Verification items for the finished model (mm, model axes). Round coordinates to 2 decimals unless told otherwise and drop trailing zeros. Write each loop counter-clockwise with the first axis right and the second up, starting at its lowest first coordinate (ties: lowest second). Pieces come first, ordered by that corner, then holes. Notation, with made-up numbers: (4.5, -22) - (31.5, -22) arc R16 ccw to (31.5, -4) - close; hole circle Ø8 at (-13, 89.25). An arc over 180 degrees is marked (long way). Answer as a JSON object with one key per item and string values.
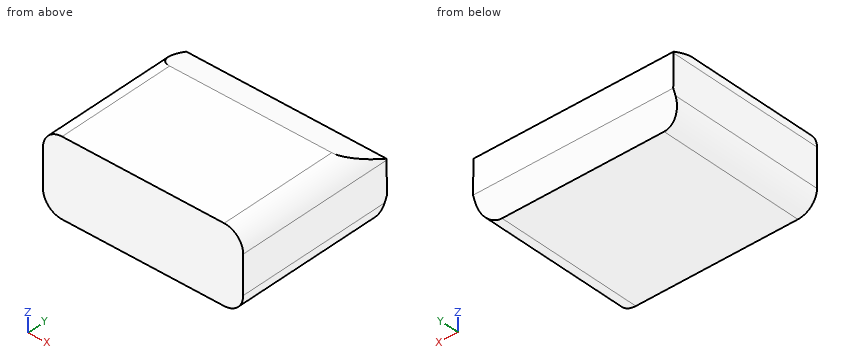
```python
from build123d import *

# Parameters (mm, degrees)
SKETCH1_W           = 105
SKETCH1_H           = 90
BOSS_EXTRUDE1_DEPTH = 40
FILLET5_R           = 10.000000066
FILLET6_R           = 10.000000066
FILLET7_R           = 10.000000066
FILLET8_R           = 10.000000066
CHAMFER14_SIZE      = 27.54
CHAMFER14_SIZE_2    = 12.3
CHAMFER15_SIZE      = 415.05734945
CHAMFER15_SIZE_2    = 7.46


with BuildPart() as part:
    # Sketch1 → Boss-Extrude1 (new body)
    with BuildSketch(Plane.XY):
        with Locations((7.000234735, -13.857374392)):
            Rectangle(SKETCH1_W, SKETCH1_H)
    extrude(amount=BOSS_EXTRUDE1_DEPTH)

    # Fillet5
    fillet5_edges = [part.edges().sort_by_distance(p)[0] for p in [
        (59.500234735, -13.857374392, 40),
    ]]
    fillet(fillet5_edges, radius=FILLET5_R)

    # Fillet6
    fillet6_edges = [part.edges().sort_by_distance(p)[0] for p in [
        (-45.499765265, -13.857374392, 40),
    ]]
    fillet(fillet6_edges, radius=FILLET6_R)

    # Fillet7
    fillet7_edges = [part.edges().sort_by_distance(p)[0] for p in [
        (59.500234735, -13.857374392, 0),
    ]]
    fillet(fillet7_edges, radius=FILLET7_R)

    # Fillet8
    fillet8_edges = [part.edges().sort_by_distance(p)[0] for p in [
        (-45.499765265, -13.857374392, 0),
    ]]
    fillet(fillet8_edges, radius=FILLET8_R)

    # Chamfer14
    # the kernel refuses this chamfer: 27.54, 12.3 mm, written as the material it takes off along each edge
    with BuildSketch(Plane(origin=(-106.873201315, 31.142625608, 0), x_dir=(0, 0.015735241575877565, 0.99987619342224), z_dir=(1, 0, 0))) as chamfer14_piece_1:
        Polygon((CHAMFER14_SIZE * 0.999876193422, CHAMFER14_SIZE * 0.0157352415759), (-CHAMFER14_SIZE_2 * 0.0157352415759, CHAMFER14_SIZE_2 * 0.999876193422), (0, 0), align=None)
    extrude(amount=227.7468721, mode=Mode.SUBTRACT)
    with BuildSketch(Plane(origin=(-106.873201315, 31.142625608, 40), x_dir=(0, 0.07864976650804911, -0.9969023092701859), z_dir=(1, 0, 0))) as chamfer14_piece_2:
        Polygon((CHAMFER14_SIZE_2 * 0.99690230927, -CHAMFER14_SIZE_2 * 0.078649766508), (-CHAMFER14_SIZE * 0.078649766508, -CHAMFER14_SIZE * 0.99690230927), (0, 0), align=None)
    extrude(amount=227.7468721, mode=Mode.SUBTRACT)

    # Chamfer15
    # the kernel refuses this chamfer: 415.05734945, 7.46 mm, written as the material it takes off along each edge
    with BuildSketch(Plane(origin=(-1124.643578574, 31.142625608, 27.7), x_dir=(0, 0.0006265203958835344, -0.9999998037360776), z_dir=(1, 0, 0))) as chamfer15_piece_1:
        Polygon((CHAMFER15_SIZE * 0.999999803737, -CHAMFER15_SIZE * 0.000626520395884), (-CHAMFER15_SIZE_2 * 0.408370910279, -CHAMFER15_SIZE_2 * 0.912816082044), (0, 0), align=None)
    extrude(amount=2263.287626617, mode=Mode.SUBTRACT)


solid = part.part
```
1. Cross-section at C-C (z = 5). Record the boundary of the cut face in (x, y).
Completed:
{"outline": "(-44.16, -58.86) - (58.16, -58.86) - (58.16, 21.08) - (-44.16, 21.08) - close"}
2. Go/stop test with a flat-tipped pin: pin 1 (2 mm diameter, centred on y = -39.5, z = 5.5, fed in from +X). Record where the tip stops, or that it passes through.
Completed:
{"pin 1": "stops at x = 58.87"}
3. Cross-section at B-B (x = 39). Record the boundary of the cut face in (y, z), plus the area to 3 significant figures.
Completed:
{"outline": "(-58.86, 0) - (18.84, 0) - (24.62, 12.94) - (24.33, 30.74) - (3.6, 40) - (-58.86, 40) - close", "area": "3,200 mm^2"}
4. Cross-section at A-A (y = -18). Record the boundary of the cut face in (x, z), plus the area to 3 significant figures.
Completed:
{"outline": "(-45.5, 10) arc R10 ccw to (-35.5, 0) - (49.5, 0) arc R10 ccw to (59.5, 10) - (59.5, 30) arc R10 ccw to (49.5, 40) - (-35.5, 40) arc R10 ccw to (-45.5, 30) - close", "area": "4,110 mm^2"}
5. Material ranges on probe 1 along X at (y, z) = (-22.5, 9); probe 2 along Y at (x, z) = (25.5, 30.5); probe 3 along Y at (x, z) = (1, 5), recorded low to high. Write a range as from..to.
Completed:
{"probe 1": "x = -45.45..59.45", "probe 2": "y = -58.86..24.34", "probe 3": "y = -58.86..21.08"}
6. Cross-section at D-D (y = 15.5). Record the boundary of the cut face in (x, z), plus the area to 3 significant figures.
Completed:
{"outline": "(-45.5, 10) arc R10 ccw to (-35.5, 0) - (49.5, 0) arc R10 ccw to (59.5, 10) - (59.5, 30) arc R10 ccw to (58.33, 34.69) - (-44.33, 34.69) arc R10 ccw to (-45.5, 30) - close", "area": "3,600 mm^2"}
